Input: part model. Units: mm. Frame: model coordinates. Face numbers are marked on the shaded views. Coordinates: 2 decimals unless noted, no trailing zeros. Order: outer loops, then holes, each group sorted by start corner. A loop starts at its lowest first (then second) coordinate and runs counter-clockwise, first axis right, second up. Notation, with made-up numbers: M -29,-6.5 L 26,-6.5 A30 cw 26,24.5 Z; hole C 27,0.5 d8. An arc over 180 degrees is marked long. One line per item, written item: value.
```python
from build123d import *

# Parameters (mm, degrees)
F0_W      = 150
F0_H      = 73
F1_DEPTH  = 7.873
F2_W      = 136
F2_H      = 63
F3_DEPTH  = 4.873
F4_R      = 1.25
F5_DEPTH  = 7.873
F6_R      = 1.25
F7_DEPTH  = 7.873
F8_R      = 1.25
F9_DEPTH  = 7.873
F10_R     = 1.25
F11_DEPTH = 7.873
F12_R     = 1.25
F13_DEPTH = 7.873
F14_R     = 1.25
F15_DEPTH = 7.873
F16_R     = 1.25
F17_DEPTH = 7.873
F18_R     = 1.25
F19_DEPTH = 7.873
F20_R     = 1.25
F21_DEPTH = 7.873
F22_R     = 1.25
F23_DEPTH = 7.873
F24_R     = 1.25
F25_DEPTH = 7.873
F26_R     = 1.25
F27_DEPTH = 7.873
F28_R     = 1.25
F29_DEPTH = 7.873
F30_R     = 1.25
F31_DEPTH = 7.873
F32_R     = 1.25
F33_DEPTH = 7.873
F34_R     = 1.25
F35_DEPTH = 7.873
F36_R     = 1.25
F37_DEPTH = 7.873
F38_R     = 1.25
F39_DEPTH = 7.873
F40_R     = 1.25
F41_DEPTH = 7.873
F42_R     = 1.25
F43_DEPTH = 7.873
F44_R     = 1.25
F45_DEPTH = 7.873
F46_R     = 1.25
F47_DEPTH = 7.873
F48_R     = 1.25
F49_DEPTH = 7.873
F50_R     = 1.25
F51_DEPTH = 7.873
F52_R     = 1.25
F53_DEPTH = 7.873
F54_R     = 1.25
F55_DEPTH = 7.873
F56_R     = 2
F57_DEPTH = 3
F58_R     = 2
F59_DEPTH = 3
F60_R     = 2
F61_DEPTH = 3
F62_R     = 2
F63_DEPTH = 3
F64_R     = 2
F65_DEPTH = 3
F66_R     = 2
F67_DEPTH = 3
F68_R     = 2
F69_DEPTH = 3
F70_R     = 2
F71_DEPTH = 3
F72_W     = 2.5
F72_H     = 4.873
F73_DEPTH = 63
F74_W     = 2.5
F74_H     = 6.5
F75_DEPTH = 0.623
F76_R     = 2
F77_DEPTH = 3
F79_R     = 2
F80_DEPTH = 3
F81_R     = 2
F82_DEPTH = 3
F78_R     = 2
F83_DEPTH = 3


with BuildPart() as f1:
    # F0 (on Top) → F1 (new body)
    with BuildSketch(Plane.XY):
        with Locations((75, 36.5)):
            Rectangle(F0_W, F0_H)
    extrude(amount=F1_DEPTH)

    # F2 (on Top) → F3 (cut)
    with BuildSketch(Plane.XY):
        with Locations((75, 36.5)):
            Rectangle(F2_W, F2_H)
    extrude(amount=F3_DEPTH, mode=Mode.SUBTRACT)

    # F4 (on face) → F5 (cut)
    with BuildSketch(Plane.XY.offset(7.873)):
        with Locations((2.5, 2.5)):
            Circle(F4_R)
    extrude(amount=-F5_DEPTH, mode=Mode.SUBTRACT)

    # F6 (on face) → F7 (cut)
    with BuildSketch(Plane.XY.offset(7.873)):
        with Locations((18, 2.5)):
            Circle(F6_R)
    extrude(amount=-F7_DEPTH, mode=Mode.SUBTRACT)

    # F8 (on face) → F9 (cut)
    with BuildSketch(Plane.XY.offset(7.873)):
        with Locations((34.5, 2.5)):
            Circle(F8_R)
    extrude(amount=-F9_DEPTH, mode=Mode.SUBTRACT)

    # F10 (on face) → F11 (cut)
    with BuildSketch(Plane.XY.offset(7.873)):
        with Locations((51, 2.5)):
            Circle(F10_R)
    extrude(amount=-F11_DEPTH, mode=Mode.SUBTRACT)

    # F12 (on face) → F13 (cut)
    with BuildSketch(Plane.XY.offset(7.873)):
        with Locations((67.5, 2.5)):
            Circle(F12_R)
    extrude(amount=-F13_DEPTH, mode=Mode.SUBTRACT)

    # F14 (on face) → F15 (cut)
    with BuildSketch(Plane.XY.offset(7.873)):
        with Locations((82.5, 2.5)):
            Circle(F14_R)
    extrude(amount=-F15_DEPTH, mode=Mode.SUBTRACT)

    # F16 (on face) → F17 (cut)
    with BuildSketch(Plane.XY.offset(7.873)):
        with Locations((99, 2.5)):
            Circle(F16_R)
    extrude(amount=-F17_DEPTH, mode=Mode.SUBTRACT)

    # F18 (on face) → F19 (cut)
    with BuildSketch(Plane.XY.offset(7.873)):
        with Locations((115.5, 2.5)):
            Circle(F18_R)
    extrude(amount=-F19_DEPTH, mode=Mode.SUBTRACT)

    # F20 (on face) → F21 (cut)
    with BuildSketch(Plane.XY.offset(7.873)):
        with Locations((132, 2.5)):
            Circle(F20_R)
    extrude(amount=-F21_DEPTH, mode=Mode.SUBTRACT)

    # F22 (on face) → F23 (cut)
    with BuildSketch(Plane.XY.offset(7.873)):
        with Locations((147.5, 2.5)):
            Circle(F22_R)
    extrude(amount=-F23_DEPTH, mode=Mode.SUBTRACT)

    # F24 (on face) → F25 (cut)
    with BuildSketch(Plane.XY.offset(7.873)):
        with Locations((2.5, 22)):
            Circle(F24_R)
    extrude(amount=-F25_DEPTH, mode=Mode.SUBTRACT)

    # F26 (on face) → F27 (cut)
    with BuildSketch(Plane.XY.offset(7.873)):
        with Locations((147.5, 22)):
            Circle(F26_R)
    extrude(amount=-F27_DEPTH, mode=Mode.SUBTRACT)

    # F28 (on face) → F29 (cut)
    with BuildSketch(Plane.XY.offset(7.873)):
        with Locations((147.5, 38.5)):
            Circle(F28_R)
    extrude(amount=-F29_DEPTH, mode=Mode.SUBTRACT)

    # F30 (on face) → F31 (cut)
    with BuildSketch(Plane.XY.offset(7.873)):
        with Locations((2.5, 38.5)):
            Circle(F30_R)
    extrude(amount=-F31_DEPTH, mode=Mode.SUBTRACT)

    # F32 (on face) → F33 (cut)
    with BuildSketch(Plane.XY.offset(7.873)):
        with Locations((2.5, 55)):
            Circle(F32_R)
    extrude(amount=-F33_DEPTH, mode=Mode.SUBTRACT)

    # F34 (on face) → F35 (cut)
    with BuildSketch(Plane.XY.offset(7.873)):
        with Locations((147.5, 55)):
            Circle(F34_R)
    extrude(amount=-F35_DEPTH, mode=Mode.SUBTRACT)

    # F36 (on face) → F37 (cut)
    with BuildSketch(Plane.XY.offset(7.873)):
        with Locations((2.5, 70.5)):
            Circle(F36_R)
    extrude(amount=-F37_DEPTH, mode=Mode.SUBTRACT)

    # F38 (on face) → F39 (cut)
    with BuildSketch(Plane.XY.offset(7.873)):
        with Locations((147.5, 70.5)):
            Circle(F38_R)
    extrude(amount=-F39_DEPTH, mode=Mode.SUBTRACT)

    # F40 (on face) → F41 (cut)
    with BuildSketch(Plane.XY.offset(7.873)):
        with Locations((18, 70.5)):
            Circle(F40_R)
    extrude(amount=-F41_DEPTH, mode=Mode.SUBTRACT)

    # F42 (on face) → F43 (cut)
    with BuildSketch(Plane.XY.offset(7.873)):
        with Locations((132, 70.5)):
            Circle(F42_R)
    extrude(amount=-F43_DEPTH, mode=Mode.SUBTRACT)

    # F44 (on face) → F45 (cut)
    with BuildSketch(Plane.XY.offset(7.873)):
        with Locations((34.5, 70.5)):
            Circle(F44_R)
        Circle(F44_R)
    extrude(amount=-F45_DEPTH, mode=Mode.SUBTRACT)

    # F46 (on face) → F47 (cut)
    with BuildSketch(Plane.XY.offset(7.873)):
        with Locations((115.5, 70.5)):
            Circle(F46_R)
    extrude(amount=-F47_DEPTH, mode=Mode.SUBTRACT)

    # F48 (on face) → F49 (cut)
    with BuildSketch(Plane.XY.offset(7.873)):
        with Locations((51, 70.5)):
            Circle(F48_R)
    extrude(amount=-F49_DEPTH, mode=Mode.SUBTRACT)

    # F50 (on face) → F51 (cut)
    with BuildSketch(Plane.XY.offset(7.873)):
        with Locations((67.5, 70.5)):
            Circle(F50_R)
    extrude(amount=-F51_DEPTH, mode=Mode.SUBTRACT)

    # F52 (on face) → F53 (cut)
    with BuildSketch(Plane.XY.offset(7.873)):
        with Locations((82.5, 70.5)):
            Circle(F52_R)
    extrude(amount=-F53_DEPTH, mode=Mode.SUBTRACT)

    # F54 (on face) → F55 (cut)
    with BuildSketch(Plane.XY.offset(7.873)):
        with Locations((99, 70.5)):
            Circle(F54_R)
    extrude(amount=-F55_DEPTH, mode=Mode.SUBTRACT)

    # F56 (on face) → F57 (cut)
    with BuildSketch(Plane.XY.offset(7.873)):
        with Locations((38.5, 65.1)):
            Circle(F56_R)
    extrude(amount=-F57_DEPTH, mode=Mode.SUBTRACT)

    # F58 (on face) → F59 (cut)
    with BuildSketch(Plane.XY.offset(7.873)):
        with Locations((15.8, 36.5)):
            Circle(F58_R)
    extrude(amount=-F59_DEPTH, mode=Mode.SUBTRACT)

    # F60 (on face) → F61 (cut)
    with BuildSketch(Plane.XY.offset(7.873)):
        with Locations((67.1, 36.5)):
            Circle(F60_R)
    extrude(amount=-F61_DEPTH, mode=Mode.SUBTRACT)

    # F62 (on face) → F63 (cut)
    with BuildSketch(Plane.XY.offset(7.873)):
        with Locations((111.5, 65.1)):
            Circle(F62_R)
    extrude(amount=-F63_DEPTH, mode=Mode.SUBTRACT)

    # F64 (on face) → F65 (cut)
    with BuildSketch(Plane.XY.offset(7.873)):
        with Locations((82.9, 36.5)):
            Circle(F64_R)
    extrude(amount=-F65_DEPTH, mode=Mode.SUBTRACT)

    # F66 (on face) → F67 (cut)
    with BuildSketch(Plane.XY.offset(7.873)):
        with Locations((134.2, 36.5)):
            Circle(F66_R)
    extrude(amount=-F67_DEPTH, mode=Mode.SUBTRACT)

    # F68 (on face) → F69 (cut)
    with BuildSketch(Plane.XY.offset(7.873)):
        with Locations((58.7, 22.8)):
            Circle(F68_R)
    extrude(amount=-F69_DEPTH, mode=Mode.SUBTRACT)

    # F70 (on face) → F71 (cut)
    with BuildSketch(Plane.XY.offset(7.873)):
        with Locations((91.3, 19.8)):
            Circle(F70_R)
    extrude(amount=-F71_DEPTH, mode=Mode.SUBTRACT)

    # F72 (on face) → F73 (join)
    with BuildSketch(Plane(origin=(0, 5, 0), x_dir=(-1, 0, 0), z_dir=(0, 1, 0))):
        with Locations((-75, 2.4365)):
            Rectangle(F72_W, F72_H)
    extrude(amount=F73_DEPTH)

    # F74 (on face) → F75 (cut)
    with BuildSketch(Plane(origin=(0, 0, 0), x_dir=(1, 0, 0), z_dir=(0, 0, -1))):
        with Locations((75, -36.5)):
            Rectangle(F74_W, F74_H)
    extrude(amount=-F75_DEPTH, mode=Mode.SUBTRACT)

    # F76 (on face) → F77 (cut)
    with BuildSketch(Plane(origin=(0, 0, 4.873), x_dir=(1, 0, 0), z_dir=(0, 0, -1))):
        with Locations((38.5, -13.8)):
            Circle(F76_R)
    extrude(amount=-F77_DEPTH, mode=Mode.SUBTRACT)

    # F79 (on face) → F80 (cut)
    with BuildSketch(Plane(origin=(0, 0, 4.873), x_dir=(1, 0, 0), z_dir=(0, 0, -1))):
        with Locations((111.5, -36.5)):
            Circle(F79_R)
    extrude(amount=-F80_DEPTH, mode=Mode.SUBTRACT)

    # F81 (on face) → F82 (cut)
    with BuildSketch(Plane(origin=(0, 0, 4.873), x_dir=(1, 0, 0), z_dir=(0, 0, -1))):
        with Locations((111.5, -13.8)):
            Circle(F81_R)
    extrude(amount=-F82_DEPTH, mode=Mode.SUBTRACT)

    # F78 (on face) → F83 (cut)
    with BuildSketch(Plane(origin=(0, 0, 4.873), x_dir=(1, 0, 0), z_dir=(0, 0, -1))):
        with Locations((38.5, -36.5)):
            Circle(F78_R)
    extrude(amount=-F83_DEPTH, mode=Mode.SUBTRACT)


solid = f1.part
```
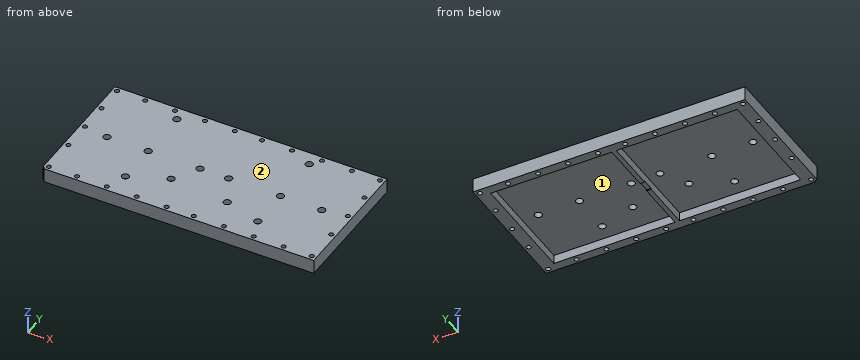
(1) Cut plane A-A on x = 91.3. Output: boundary loops of the cut face in (y, z), plus the area to 3 significant figures.
Data:
outline: M 0,0 L 5,0 L 5,4.87 L 17.8,4.87 L 17.8,7.87 L 0,7.87 Z; M 21.8,4.87 L 68,4.87 L 68,0 L 73,0 L 73,7.87 L 21.8,7.87 Z
area: 256 mm2
(2) Cut plane C-C on y = 6.5. Output: boundary loops of the cut face in (x, z).
Data:
outline: M 0,0 L 7,0 L 7,4.87 L 73.75,4.87 L 73.75,0 L 76.25,0 L 76.25,4.87 L 143,4.87 L 143,0 L 150,0 L 150,7.87 L 0,7.87 Z
(3) First-contact query: pin 1 (8 mm diameter, centred on x = 103, y = 33.5, fed in from -Z). Flat tip, straight axial feed; report the tip coordinate or a pass-through.
Data:
pin 1: stops at z = 4.87
(4) Cut plane B-B on x = 38.5. Output: boundary loops of the cut face in (y, z).
Data:
outline: M 0,0 L 5,0 L 5,4.87 L 11.8,4.87 L 11.8,7.87 L 0,7.87 Z; M 15.8,4.87 L 34.5,4.87 L 34.5,7.87 L 15.8,7.87 Z; M 38.5,4.87 L 63.1,4.87 L 63.1,7.87 L 38.5,7.87 Z; M 67.1,4.87 L 68,4.87 L 68,0 L 73,0 L 73,7.87 L 67.1,7.87 Z
(5) Ray query, line 1 (Y direction, x = 99, z = 3.75); line 2 (X direction, y = 15.5, z = 0.5); line 3 (Y direction, x = 90.5, z = 2.5). Return the intervals inside material, ascending. Write a range as from..to.
Data:
line 1: y = 0..1.25, 3.75..5, 68..69.25, 71.75..73
line 2: x = 0..7, 73.75..76.25, 143..150
line 3: y = 0..5, 68..73
(6) Draft query along Y for the marked faces 1 and 2. Return one class per face: released by +Y, released by -Y, zero draft, split by the parting line, or undercut.
Data:
face 1: undercut
face 2: zero draft
